Here's how the part is built. I have some questions about the finished solid (model axes, mm). A direction names the side the tool comes from. Give positions to 0.01 mm unless a question says otherwise; leave off trailing zeros. Loops run counter-clockwise (first coordinate to the right, second up) from the corner with the lowest first, then second, coordinate; pieces in that order, holes last. Notation, with made-up numbers: M -21,87.5 L 5,87.5 A27 cw 5,113.5 Z; hole C 68,34.25 d8. An arc over 180 degrees is marked long. Answer as CSV lines item,"result". Start each with the question number.
Item 1: For faces 1 (the flat face through (40, 20, 20)), 2 (the flat face through (20, 30, 24)), which set-ups out of +Z, -Z, +X, -X, +Y, -Y let a thin tool reach every point of the face, with its end or its side?
Item 2: I want a section at D-D on x = 16.5. List the corners of the cut face in (y, z) for me, plus the area to 3 significant figures.
Item 3: Will these pins go through, and if not, where does the flat tip stop? P1, Ø3, axis at x = 18, z = 26.5, coming from the +Y side; P2, Ø1, axis at x = 7, z = 31.5, coming from the -Y side; P3, Ø6, axis at y = 33, z = 12.5, coming from the -X side.
Item 4: I want a section at C-C on y = 7. List the corners of the cut face in (x, z) for me, plus the area to 3 significant figures.
Item 5: I want a section at A-A on z = 34. List the corners of the cut face in (x, y) for me, plus the area to 3 significant figures.
Item 6: I want a section at B-B on x = 29.5. List the corners of the cut face in (y, z) for me.
Item 7: If I drill on line 1 along X through (y, z) = (33.5, 22); line 2 along Y through (x, z) = (18, 12); line 3 along Y through (x, z) = (22, 3), over which ranges is the centre line in solid material (lowest first)? Write a range as from..to.
from build123d import *

# Parameters (mm, degrees)
SKETCH1_W           = 40
SKETCH1_H           = 20
BOSS_EXTRUDE1_DEPTH = 40
CUT_EXTRUDE1_DEPTH  = 40
SKETCH4_W           = 20
SKETCH4_H           = 20
BOSS_EXTRUDE3_DEPTH = 40
CUT_EXTRUDE2_DEPTH  = 40


with BuildPart() as part:
    # Sketch1 → Boss-Extrude1 (new body)
    with BuildSketch(Plane.XY):
        with Locations((20, 10)):
            Rectangle(SKETCH1_W, SKETCH1_H)
    extrude(amount=BOSS_EXTRUDE1_DEPTH)

    # Sketch2 → Cut-Extrude1 (cut)
    with BuildSketch(Plane.ZY):
        Polygon((40, 20), (20, 0), (40, 0), align=None)
    extrude(amount=-CUT_EXTRUDE1_DEPTH, mode=Mode.SUBTRACT)

    # Sketch4 → Boss-Extrude3 (add)
    with BuildSketch(Plane(origin=(0, 0, 0), x_dir=(-1, 0, 0), z_dir=(0, 0, -1))):
        with Locations((-30, 30)):
            Rectangle(SKETCH4_W, SKETCH4_H)
    extrude(amount=-BOSS_EXTRUDE3_DEPTH)

    # Sketch5 → Cut-Extrude2 (cut)
    with BuildSketch(Plane.ZY.offset(-20)):
        Polygon((0, 20), (20, 40), (0, 40), align=None)
    extrude(amount=-CUT_EXTRUDE2_DEPTH, mode=Mode.SUBTRACT)


solid = part.part
Result:
1,face 1,"+Z, -Z, +X, +Y, -Y"
1,face 2,"+Z, -Z, -X, +Y"
2,outline,"M 0,0 L 20,0 L 20,40 L 0,20 Z"
2,area,"600 mm^2"
3,P1,"y = 20"
3,P2,"y = 11"
3,P3,"x = 20"
4,outline,"M 0,0 L 40,0 L 40,27 L 0,27 Z"
4,area,"1,080 mm^2"
5,outline,"M 0,14 L 40,14 L 40,40 L 20,40 L 20,20 L 0,20 Z"
5,area,"640 mm^2"
6,outline,"M 0,0 L 20,0 L 40,20 L 40,40 L 20,40 L 0,20 Z"
7,line 1,"20..40"
7,line 2,"0..20"
7,line 3,"0..23"
